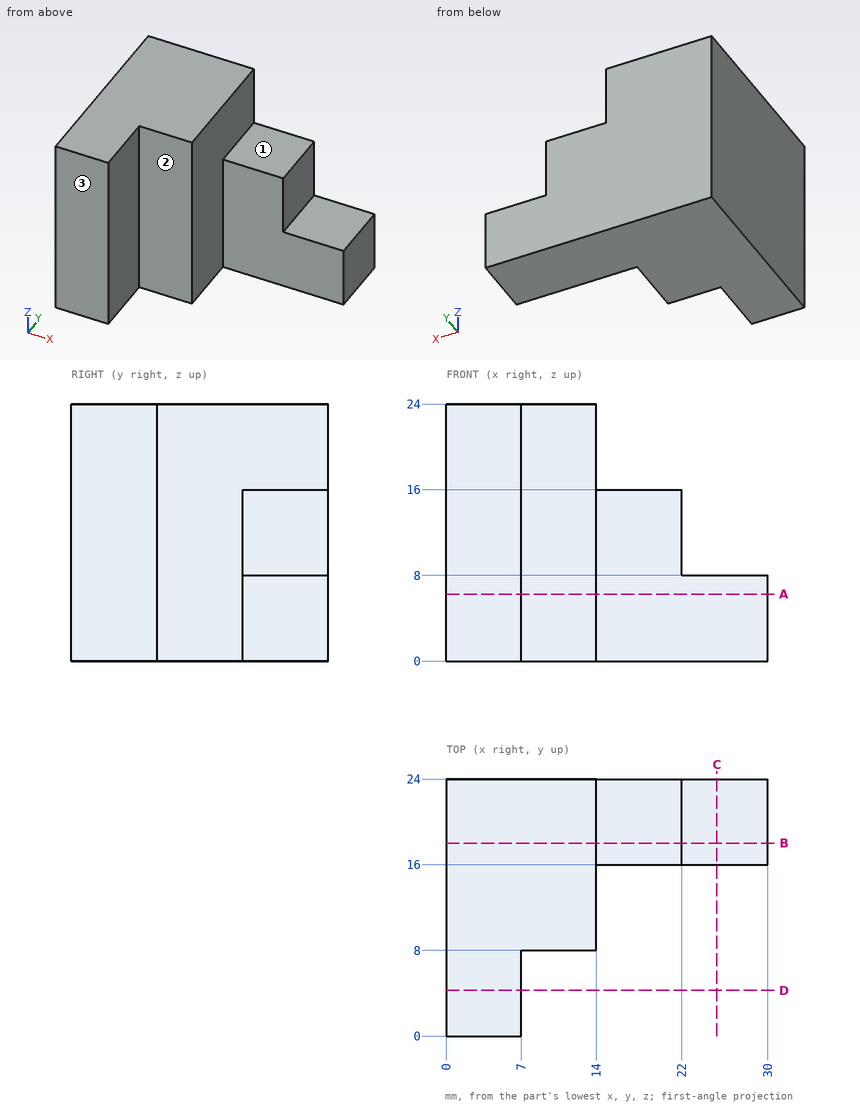
The drawing under review shows one solid part. Ordinate dimensions are in mm from its lowest x, y, z. A direction names the side the tool comes from. Coordinates: 2 decimals unless noted, no trailing zeros. Loops run counter-clockwise (first coordinate to the right, second up) from the corner with the lowest first, then second, coordinate; pieces in that order, holes last. Notation, with made-up numbers: M 77.5,-15.75 L 123.5,-15.75 A18 cw 123.5,8.25 Z; hole C 3,-23.75 d7. An arc over 180 degrees is marked long. Use one line per item in the form item = value.
(1) For the marked faces 1, 2 and 3, list the 3-axis set-ups (+Z, -Z, +X, -X, +Y, -Y) from which the entire face can be reached by the end or side of a thin tool; tool diameter is ignored.
Return value:
face_1 = +Z, +X, +Y, -Y
face_2 = +Z, -Z, +X, -Y
face_3 = +Z, -Z, +X, -X, -Y
(2) Consider section A-A (z = 6.25). Write out the cut boundary in (x, y), and give its area (3 significant figures).
Return value:
outline = M 0,0 L 7,0 L 7,8 L 14,8 L 14,16 L 30,16 L 30,24 L 0,24 Z
area = 408 mm2
(3) Consider section C-C (x = 25.25). Write out the cut boundary in (y, z).
Return value:
outline = M 16,0 L 24,0 L 24,8 L 16,8 Z
(4) Clearance check with flat-ended pins moving along their axes: P1, Ø6.5, axis at x = 26.5, y = 19, coming from the +Z side; P2, Ø4, axis at y = 4.5, z = 7.5, coming from the +X side; P3, Ø5, axis at x = 22.5, z = 10, coming from the -Y side. State where each tip first meets the part, or that it passes through.
Return value:
P1 = 8
P2 = 7
P3 = 16
(5) For line 1 along Y through (x, z) = (21.75, 7.5); line 2 along X through (y, z) = (8.25, 13.5); line 3 along X through (y, z) = (2, 21.25), list the stretches that pass through material, from the lowest coordinate up. Write a range as from..to.
Return value:
line_1 = 16..24
line_2 = 0..14
line_3 = 0..7
(6) Consider section B-B (y = 18). Write out the cut boundary in (x, z).
Return value:
outline = M 0,0 L 30,0 L 30,8 L 22,8 L 22,16 L 14,16 L 14,24 L 0,24 Z
(7) Consider section D-D (y = 4.25). Write out the cut boundary in (x, z), and give its area (3 significant figures).
Return value:
outline = M 0,0 L 7,0 L 7,24 L 0,24 Z
area = 168 mm2
